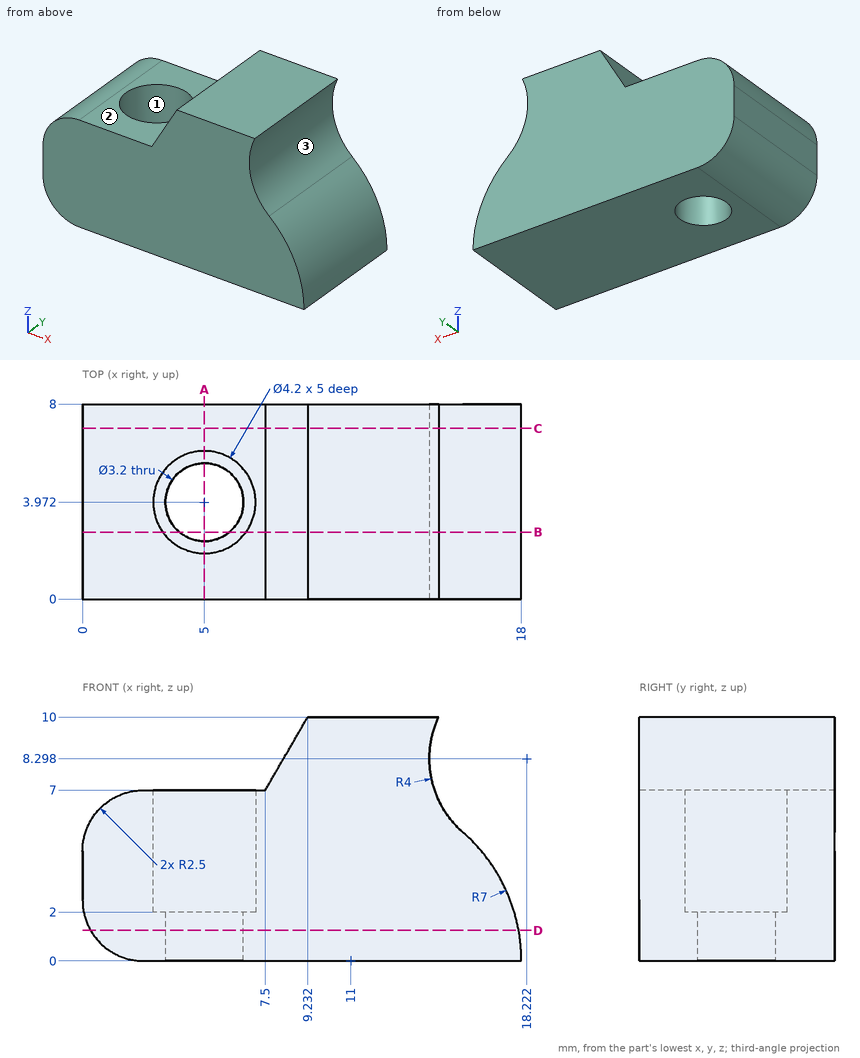
Here's the drawing with two shaded views (mm, measured from the low corner). I have some questions. Give positions to 0.01 mm unless a question says otherwise; leave off trailing zeros. Order: outer loops, then holes, each group sorted by start corner. A loop starts at its lowest first (then second) coordinate and runs counter-clockwise, first axis right, second up. Notation, with made-up numbers: M -13,-0.5 L 32,-0.5 A30 cw 32,35.5 Z; hole C -13.75,67.25 d10. An arc over 180 degrees is marked long. One line per question, with ' | ' between items.
Item 1: Suppose I cut it at C-C, the plane y = 7. Write out the boundary of the cut face in (x, z) (1 decimal), then the cut area to 3 significant figures.
Answer block:
outline: M 0,2.5 A2.5 ccw 2.5,0 L 18,0 A7 ccw 15.6,5.3 A4 cw 14.6,10 L 9.2,10 L 7.5,7 L 2.5,7 A2.5 ccw 0,4.5 Z | area: 132 mm2
Item 2: Please list where these lines run through material, in increasing order: L1, parallel to Y at x = 5, z = 3.7; L2, parallel to Y at x = 5, z = 0.5; L3, parallel to Z at x = 3.5, y = 6.25.
Answer block:
L1: y = 0 to 1.87, 6.07 to 8 | L2: y = 0 to 2.37, 5.57 to 8 | L3: z = 0 to 7
Item 3: We'd pull the mould along X, two halves only. Please class the marked faces 1, 2 and 3: released by +X, released by -X, zero draft, split by the parting line, or undercut.
Answer block:
face 1: undercut | face 2: zero draft | face 3: released by +X
Item 4: Suppose I cut it at D-D, the plane z = 1.25. Write out the boundary of the cut face in (x, y) (1 decimal).
Answer block:
outline: M 0.3,0 L 17.9,0 L 17.9,8 L 0.3,8 Z; hole C 5,4 d3.2
Item 5: Suppose I cut it at A-A, the plane x = 5. Write out the boundary of the cut face in (y, z).
Answer block:
outline: M 0,0 L 2.37,0 L 2.37,2 L 1.87,2 L 1.87,7 L 0,7 Z; M 5.57,0 L 8,0 L 8,7 L 6.07,7 L 6.07,2 L 5.57,2 Z
Item 6: I'm going to push flat-ended pins straight in: pin 1 Ø3 at (y, z) = (1, 7) entering from +X; pin 2 Ø1.3 at (x, y) = (4, 4) entering from +Z; pin 3 Ø3 at (y, z) = (6, 3.5) entering from -X; pin 4 Ø1 at (y, z) = (6, 9) entering from +X. Where does each tip first touch, or does it pass through?
Answer block:
pin 1: stops at x = 15.36 | pin 2: stops at z = 2 | pin 3: stops at x = 0 | pin 4: stops at x = 14.41
Item 7: Suppose I cut it at B-B, the plane y = 2.75. Write out the boundary of the cut face in (x, z) (1 decimal).
Answer block:
outline: M 0,2.5 A2.5 ccw 2.5,0 L 4,0 L 4,2 L 3.3,2 L 3.3,7 L 2.5,7 A2.5 ccw 0,4.5 Z; M 6,0 L 18,0 A7 ccw 15.6,5.3 A4 cw 14.6,10 L 9.2,10 L 7.5,7 L 6.7,7 L 6.7,2 L 6,2 Z
